CAD build for the part. Positions are in the model's coordinates, mm. Give positions to 0.01 mm unless a question says otherwise; leave off trailing zeros. Order: outer loops, then holes, each group sorted by start corner. A loop starts at its lowest first (then second) coordinate and runs counter-clockwise, first axis right, second up. Notation, with made-up numbers: (49.25, 1) -> (63.25, 1) arc R24 cw to (63.25, 19) -> close; hole circle Ø10 at (-29, 84.25). An arc over 180 degrees is marked (long way). Use one line per item in the form item = value. Start each with the question number.
1) Cut at C-C, the plane z = 17.5. Give the cut face in (x, y).
2) Cut at D-D, the plane y = 82.5. Give the cut face in (x, z).
3) Cut at A-A, the plane y = 0. Give the cut face in (x, z).
4) Cut at B-B, the plane x = 0. Give the cut face in (y, z).
5) Drop flat-ended pins along their axis: P1, Ø15.5, axis at x = 120, y = 82.5, coming from the +Z side; P2, Ø12, axis at x = -120, y = 82.5, coming from the -Z side. Give the stop position or say it passes through.
6) Probe line 1 (X direction, y = -82, z = 46); line 2 (X direction, y = -82, z = 24); line 3 (Y direction, x = -65, z = 21). List the from-to ranges inside material, lowest first.
from build123d import *

# Parameters (mm, degrees)
SKETCH1_W           = 280
SKETCH1_H           = 245
SKETCH1_R           = 15
SKETCH1_R_2         = 5.25
BOSS_EXTRUDE1_DEPTH = 50
SKETCH2_R           = 8.5
CUT_EXTRUDE1_DEPTH  = 12


with BuildPart() as part:
    # Sketch1 → Boss-Extrude1 (new body)
    with BuildSketch(Plane.XY):
        Rectangle(SKETCH1_W, SKETCH1_H)
        Circle(SKETCH1_R, mode=Mode.SUBTRACT)
        with Locations((-120, 82.5)):
            Circle(SKETCH1_R_2, mode=Mode.SUBTRACT)
        with Locations((120, 82.5)):
            Circle(SKETCH1_R_2, mode=Mode.SUBTRACT)
        with Locations((-65, -82.5)):
            Circle(SKETCH1_R_2, mode=Mode.SUBTRACT)
        with Locations((65, -82.5)):
            Circle(SKETCH1_R_2, mode=Mode.SUBTRACT)
    extrude(amount=BOSS_EXTRUDE1_DEPTH)

    # Sketch2 → Cut-Extrude1 (cut)
    with BuildSketch(Plane.XY.offset(50)):
        with Locations((-120, 82.5)):
            Circle(SKETCH2_R)
        with Locations((120, 82.5)):
            Circle(SKETCH2_R)
        with Locations((65, -82.5)):
            Circle(SKETCH2_R)
        with Locations((-65, -82.5)):
            Circle(SKETCH2_R)
    extrude(amount=-CUT_EXTRUDE1_DEPTH, mode=Mode.SUBTRACT)


solid = part.part
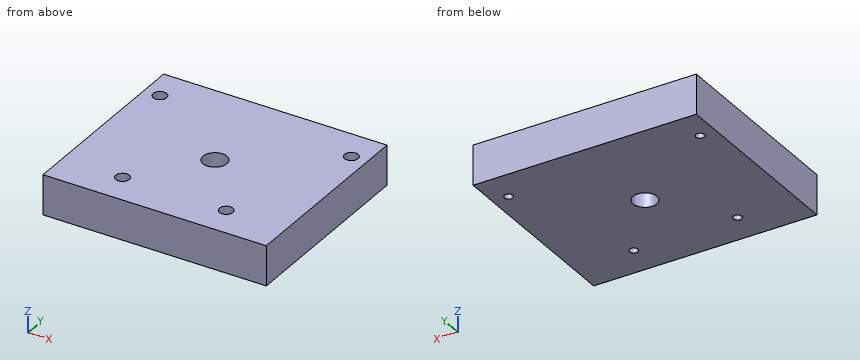
Result:
q1.outline = (-140, -122.5) -> (140, -122.5) -> (140, 122.5) -> (-140, 122.5) -> close; hole circle Ø10.5 at (-120, 82.5); hole circle Ø10.5 at (-65, -82.5); hole circle Ø30 at (0, 0); hole circle Ø10.5 at (65, -82.5); hole circle Ø10.5 at (120, 82.5)
q2.outline = (-140, 0) -> (-125.25, 0) -> (-125.25, 38) -> (-128.5, 38) -> (-128.5, 50) -> (-140, 50) -> close; (-114.75, 0) -> (114.75, 0) -> (114.75, 38) -> (111.5, 38) -> (111.5, 50) -> (-111.5, 50) -> (-111.5, 38) -> (-114.75, 38) -> close; (125.25, 0) -> (140, 0) -> (140, 50) -> (128.5, 50) -> (128.5, 38) -> (125.25, 38) -> close
q3.outline = (-140, 0) -> (-15, 0) -> (-15, 50) -> (-140, 50) -> close; (15, 0) -> (140, 0) -> (140, 50) -> (15, 50) -> close
q4.outline = (-122.5, 0) -> (-15, 0) -> (-15, 50) -> (-122.5, 50) -> close; (15, 0) -> (122.5, 0) -> (122.5, 50) -> (15, 50) -> close
q5.P1 = 38
q5.P2 = 0
q6.line_1 = -140 to -73.49, -56.51 to 56.51, 73.49 to 140
q6.line_2 = -140 to -70.23, -59.77 to 59.77, 70.23 to 140
q6.line_3 = -122.5 to -87.75, -77.25 to 122.5
